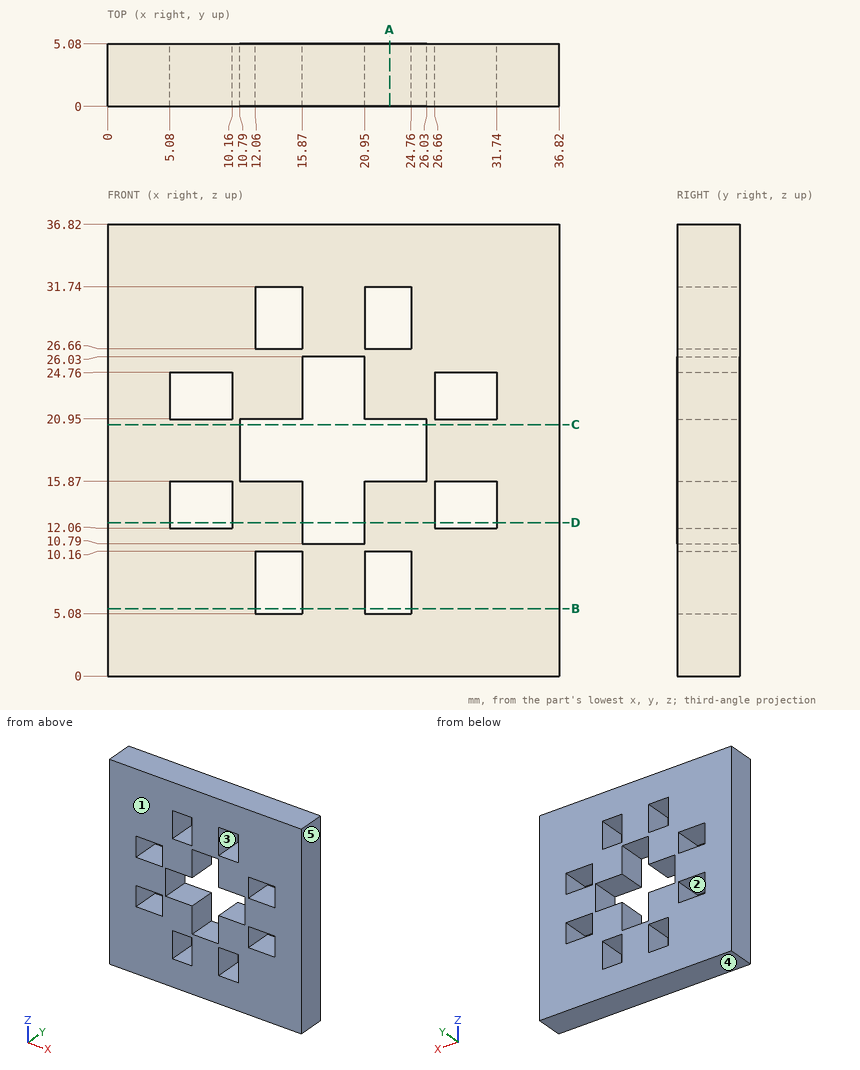
Study the drawing (mm; zero at the part's minimum x, y, z) and answer. A direction names the side the tool comes from. Give positions to 0.01 mm unless a question says otherwise; leave off trailing zeros. Order: outer loops, then holes, each group sorted by start corner. A loop starts at its lowest first (then second) coordinate and runs counter-clockwise, first axis right, second up. Notation, with made-up numbers: (47, 24.25) -> (92, 24.25) arc R27 ccw to (92, 56.25) -> close; hole circle Ø7 at (20.5, 54.5). An arc over 180 degrees is marked (long way). Put each result on its own line as item: value.
Item 1: A cutting plane is placed at D-D on z = 12.5. Give the vertices of the cut face in (x, y).
Established:
outline: (0, 0) -> (5.08, 0) -> (5.08, 5.08) -> (0, 5.08) -> close; (10.16, 0) -> (15.87, 0) -> (15.87, 5.08) -> (10.16, 5.08) -> close; (20.95, 0) -> (26.66, 0) -> (26.66, 5.08) -> (20.95, 5.08) -> close; (31.74, 0) -> (36.82, 0) -> (36.82, 5.08) -> (31.74, 5.08) -> close
Item 2: Straight lines are drawn through the part: line 1 (Z direction, x = 30.5, y = 2.35); line 2 (Z direction, x = 15.5, y = 2.5). For each, find the intervals that lie inside material, in ascending order.
Established:
line 1: z = 0 to 12.06, 15.87 to 20.95, 24.76 to 36.82
line 2: z = 0 to 5.08, 10.16 to 15.87, 20.95 to 26.66, 31.74 to 36.82
Item 3: A cutting plane is placed at C-C on z = 20.5. Give the vertices of the cut face in (x, y).
Established:
outline: (0, 0) -> (10.79, 0) -> (10.79, 5.08) -> (0, 5.08) -> close; (26.03, 0) -> (36.82, 0) -> (36.82, 5.08) -> (26.03, 5.08) -> close
Item 4: For the marked faces 1 and 2, determine the directions among +Z, -Z, +X, -X, +Y, -Y from which every point of the face is accessible in a straight line to the end or side of a thin tool.
Established:
face 1: +Z, -Z, +X, -X, -Y
face 2: +Y, -Y
Item 5: For a pull along X with two mould halves and no side action, classify the marked faces 3, 4 and 5 as released by +X, released by -X, zero draft, split by the parting line, or undercut.
Established:
face 3: undercut
face 4: zero draft
face 5: released by +X
Item 6: A cutting plane is placed at B-B on z = 5.5. Give the vertices of the cut face in (x, y).
Established:
outline: (0, 0) -> (12.06, 0) -> (12.06, 5.08) -> (0, 5.08) -> close; (15.87, 0) -> (20.95, 0) -> (20.95, 5.08) -> (15.87, 5.08) -> close; (24.76, 0) -> (36.82, 0) -> (36.82, 5.08) -> (24.76, 5.08) -> close
Item 7: A cutting plane is placed at A-A on x = 23. Give the vertices of the cut face in (y, z), plus the area to 3 significant figures.
Established:
outline: (0, 0) -> (5.08, 0) -> (5.08, 5.08) -> (0, 5.08) -> close; (0, 10.16) -> (5.08, 10.16) -> (5.08, 15.87) -> (0, 15.87) -> close; (0, 20.95) -> (5.08, 20.95) -> (5.08, 26.66) -> (0, 26.66) -> close; (0, 31.74) -> (5.08, 31.74) -> (5.08, 36.82) -> (0, 36.82) -> close
area: 110 mm^2
